```python
from build123d import *

# Parameters (mm, degrees)
SALIENTE_EXTRUIR1_DEPTH = 65.5
CROQUIS2_R              = 3
CORTAR_EXTRUIR1_DEPTH   = 20
CROQUIS3_R              = 6
CORTAR_EXTRUIR2_DEPTH   = 20
CROQUIS4_R              = 4.5
CORTAR_EXTRUIR3_DEPTH   = 6


with BuildPart() as part:
    # Croquis1 → Saliente-Extruir1 (new body)
    with BuildSketch(Plane.XY):
        with BuildLine():
            Line((-15, -30), (-15, -33.5))
            Line((-15, -33.5), (15, -33.5))
            Line((15, -33.5), (15, -30))
            Line((15, -30), (21, -30))
            ThreePointArc((21, -30), (27.363961031, -27.363961031), (30, -21))
            Line((30, -21), (30, 21))
            ThreePointArc((30, 21), (27.363961031, 27.363961031), (21, 30))
            Line((21, 30), (-21, 30))
            ThreePointArc((-21, 30), (-27.363961031, 27.363961031), (-30, 21))
            Line((-30, 21), (-30, -21))
            ThreePointArc((-30, -21), (-27.363961031, -27.363961031), (-21, -30))
            Line((-21, -30), (-15, -30))
        make_face()
    extrude(amount=-SALIENTE_EXTRUIR1_DEPTH)

    # Croquis2 → Cortar-Extruir1 (cut)
    with BuildSketch(Plane.XY):
        with Locations((-21, 21)):
            Circle(CROQUIS2_R)
        with Locations((21, 21)):
            Circle(CROQUIS2_R)
        with Locations((21, -21)):
            Circle(CROQUIS2_R)
        with Locations((-21, -21)):
            Circle(CROQUIS2_R)
    extrude(amount=-CORTAR_EXTRUIR1_DEPTH, mode=Mode.SUBTRACT)

    # Croquis3 → Cortar-Extruir2 (cut)
    with BuildSketch(Plane.XY):
        Circle(CROQUIS3_R)
    extrude(amount=-CORTAR_EXTRUIR2_DEPTH, mode=Mode.SUBTRACT)

    # Croquis4 → Cortar-Extruir3 (cut)
    with BuildSketch(Plane.XZ.offset(33.5)):
        with Locations(Location((0, -5.5, 0), (0, 0, 270))):
            Circle(CROQUIS4_R)
        with Locations(Location((0, -60, 0), (0, 0, 270))):
            Circle(CROQUIS4_R)
    extrude(amount=-CORTAR_EXTRUIR3_DEPTH, mode=Mode.SUBTRACT)


solid = part.part
```
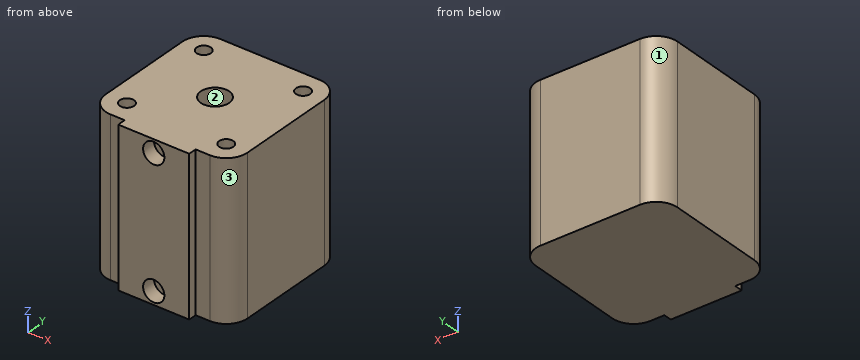
Model file for the job. Use its own axes, mm. Face numbers are marked on the shaded views. Give positions to 0.01 mm unless a question says otherwise; leave off trailing zeros. Write each loop counter-clockwise with the first axis right and the second up, starting at its lowest first coordinate (ties: lowest second). Pieces come first, ordered by that corner, then holes. Notation, with made-up numbers: (-1, 8.5) - (16, 8.5) arc R30 cw to (16, 35.5) - close; hole circle Ø11 at (46, -19.5). An arc over 180 degrees is marked (long way). One line per question, with ' | ' between items. Start each with the question number.
(1) Pin check, flat tips, straight feed: P1, Ø3, axis at x = 21, y = 21, coming from the +Z side; P2, Ø1.8, axis at x = -17, z = -41, coming from the -Y side; P3, Ø8, axis at y = -26, z = -47, coming from the +X side. Stop position of each tip, or through.
(2) Slice it at B-B on z = -60. Write the cut outline in (x, y).
(3) Wall check: line 1 along Y through (x, z) = (-21, -8.25); line 2 along Y through (x, z) = (0, -7.25); line 3 along X through (y, z) = (2, -2.5). Give the ranges that are in metal, low to high. Write a range as from..to.
(4) Slice it at D-D on z = -14.5. Write the cut outline in (x, y), plus the area to 3 significant figures.
(5) Slice it at A-A on y = 0. Write the cut outline in (x, z), plus the area to 3 significant figures.
(6) Two-plate mould, pull along X, no slides. Class the marked faces 1, 2 and 3: +X half, -X half, draft (parallel to the pull), parting line (faces both ways), or undercut.
(7) Slice it at C-C on x = 0. Write the cut outline in (y, z), plus the area to 3 significant figures.
Results below:
1) P1: z = -20 | P2: y = -30 | P3: x = 29.94
2) outline: (-30, -21) arc R9 ccw to (-21, -30) - (-15, -30) - (-15, -33.5) - (-4.5, -33.5) - (-4.5, -27.5) - (4.5, -27.5) - (4.5, -33.5) - (15, -33.5) - (15, -30) - (21, -30) arc R9 ccw to (30, -21) - (30, 21) arc R9 ccw to (21, 30) - (-21, 30) arc R9 ccw to (-30, 21) - close
3) line 1: -30..-24, -18..18, 24..30 | line 2: -27.5..-6, 6..30 | line 3: -30..-5.66, 5.66..30
4) outline: (-30, -21) arc R9 ccw to (-21, -30) - (-15, -30) - (-15, -33.5) - (15, -33.5) - (15, -30) - (21, -30) arc R9 ccw to (30, -21) - (30, 21) arc R9 ccw to (21, 30) - (-21, 30) arc R9 ccw to (-30, 21) - close; hole circle Ø6 at (-21, -21); hole circle Ø6 at (-21, 21); hole circle Ø12 at (0, 0); hole circle Ø6 at (21, -21); hole circle Ø6 at (21, 21) | area: 3,410 mm^2
5) outline: (-30, -65.5) - (30, -65.5) - (30, 0) - (6, 0) - (6, -20) - (-6, -20) - (-6, 0) - (-30, 0) - close | area: 3,690 mm^2
6) face 1: -X half | face 2: undercut | face 3: +X half
7) outline: (-33.5, -65.5) - (30, -65.5) - (30, 0) - (6, 0) - (6, -20) - (-6, -20) - (-6, 0) - (-33.5, 0) - (-33.5, -1) - (-27.5, -1) - (-27.5, -10) - (-33.5, -10) - (-33.5, -55.5) - (-27.5, -55.5) - (-27.5, -64.5) - (-33.5, -64.5) - close | area: 3,810 mm^2
